Source: CAD feature listing. Evaluate the final solid. Frame: model axes, mm. A direction names the side the tool comes from. Round coordinates to 2 decimals unless told otherwise and drop trailing zeros. Write each loop counter-clockwise with the first axis right and the second up, starting at its lowest first coordinate (ties: lowest second). Pieces come first, ordered by that corner, then holes.
from build123d import *

# Parameters (mm, degrees)
F0_R      = 7.5
F1_DEPTH  = 14
F4_R      = 1.5
F5_DEPTH  = 15.001
F6_R      = 1.1
F7_DEPTH  = 5
F9_DEPTH  = 5
F13_DEPTH = 15.0010001


with BuildPart() as f1:
    # F0 (on Top) → F1 (new body)
    with BuildSketch(Plane.XY):
        Circle(F0_R)
    extrude(amount=F1_DEPTH)

    # F4 (on line) → F5 (cut, through all)
    with BuildSketch(Plane(origin=(0, 7.5, 0), x_dir=(-1, 0, 0), z_dir=(0, 1, 0))):
        with Locations((0, 3.7)):
            Circle(F4_R)
    extrude(amount=-F5_DEPTH, mode=Mode.SUBTRACT)

    # F6 (on face) → F7 (cut)
    with BuildSketch(Plane.XY.offset(14)):
        Circle(F6_R)
    extrude(amount=-F7_DEPTH, mode=Mode.SUBTRACT)

    # F8 (on face) → F9 (cut, through all)
    with BuildSketch(Plane.XY.offset(14)):
        with BuildLine():
            ThreePointArc((-7.5, 0), (-7.4962990893, -0.2355843037), (-7.4852000096, -0.470936107))
            Line((-7.4852000096, -0.470936107), (-0.9940921402, -0.470936107))
            ThreePointArc((-0.9940921402, -0.470936107), (-1.1, 0), (-0.9940921402, 0.470936107))
            Line((-0.9940921402, 0.470936107), (-7.4852000096, 0.470936107))
            ThreePointArc((-7.4852000096, 0.470936107), (-7.4962990893, 0.2355843037), (-7.5, 0))
        make_face()
        with BuildLine():
            Line((0.9940921402, -0.470936107), (7.4852000096, -0.470936107))
            ThreePointArc((7.4852000096, -0.470936107), (7.4962990893, -0.2355843037), (7.5, 0))
            ThreePointArc((7.5, 0), (7.4962990893, 0.2355843037), (7.4852000096, 0.470936107))
            Line((7.4852000096, 0.470936107), (0.9940921402, 0.470936107))
            ThreePointArc((0.9940921402, 0.470936107), (1.0731964765, 0.241348965), (1.1, 0))
            ThreePointArc((1.1, 0), (1.0731964765, -0.241348965), (0.9940921402, -0.470936107))
        make_face()
    extrude(amount=-F9_DEPTH, mode=Mode.SUBTRACT)

    # F12 (on line) → F13 (cut, through all)
    with BuildSketch(Plane.YZ.offset(-7.5)):
        Polygon((-0.9654102032, 9), (-0.470936107, 9), (0.470936107, 9), (0.9545897968, 9), (0.9545897968, 10.92), (-0.9654102032, 10.92), align=None)
    extrude(amount=F13_DEPTH, mode=Mode.SUBTRACT)


solid = f1.part
1) Contact query for flat-ended pins moving along their axis: P1, Ø1, axis at y = -6, z = 5, coming from the -X side; P2, Ø0.6, axis at x = 5, z = 10.5, coming from the +Y side; P3, Ø1.5, axis at y = 5, z = 3, coming from the -X side. Output: stop coordinate, or through.
Taken from the geometry:
P1: stops at x = -5.1
P2: stops at y = 5.84
P3: stops at x = -6.18
2) Reachability of faces 1 (the face through (0, 1.1, 12.1)), 2 (the face through (4, 0.471, 12)), 3 (the face through (4, -0.965, 10)), 4 (the face through (0.195, 0.103, 5.187)) from +Z, -Z, +X, -X, +Y, -Y: full face, straight path, thin tool, end or side. Return the list, or none.
Taken from the geometry:
face 1: +Z
face 2: +Z, +X, -X
face 3: +X, -X
face 4: +Y, -Y
3) Section query C-C on y = 0. Return the cut outline in (x, z).
Taken from the geometry:
outline: (-7.5, 0) - (7.5, 0) - (7.5, 9) - (-7.5, 9) - close; hole circle Ø3 at (0, 3.7)
4) Material intervals for line 1 (Z direction, x = 0, y = -0.5); line 2 (Z direction, x = 0, y = 4); line 3 (X direction, y = 0.25, z = 3.7), sorted ascending.
Taken from the geometry:
line 1: z = 0 to 2.2, 5.2 to 9
line 2: z = 0 to 2.2, 5.2 to 14
line 3: x = -7.5 to -1.5, 1.5 to 7.5
5) Pull-direction query (Z, two-part tool) for faces 5 (the face through (4, 0.955, 10)), 6 (the face through (0, 3, 14)), 7 (the face through (0, 0, 0)), 8 (the face through (-4, 0.471, 12)); classes: released by +Z, released by -Z, zero draft, split by the parting line, or undercut.
Taken from the geometry:
face 5: undercut
face 6: released by +Z
face 7: released by -Z
face 8: zero draft
6) Section query D-D on x = -5.25. Return the cut outline in (y, z).
Taken from the geometry:
outline: (-5.36, 0) - (5.36, 0) - (5.36, 14) - (0.47, 14) - (0.47, 10.92) - (0.95, 10.92) - (0.95, 9) - (-0.97, 9) - (-0.97, 10.92) - (-0.47, 10.92) - (-0.47, 14) - (-5.36, 14) - close
7) Section query B-B on x = 0. Return the cut outline in (y, z), then the cut area to 3 significant figures.
Taken from the geometry:
outline: (-7.5, 0) - (7.5, 0) - (7.5, 2.2) - (-7.5, 2.2) - close; (-7.5, 5.2) - (7.5, 5.2) - (7.5, 14) - (1.1, 14) - (1.1, 9) - (-1.1, 9) - (-1.1, 14) - (-7.5, 14) - close
area: 154 mm2
